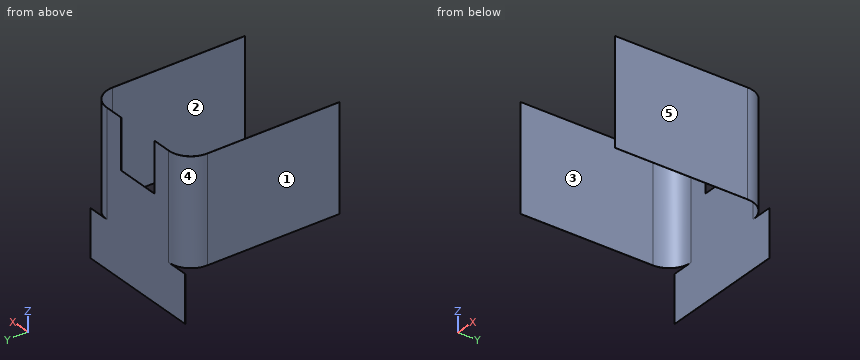
```python
from build123d import *

# Parameters (mm, degrees)
F1_DEPTH = 380
F2_W     = 80
F2_H     = 180
F2_H_2   = 115.651754
F3_DEPTH = 25.4
F4_W     = 230
F4_H     = 170
F5_DEPTH = 0.6


with BuildPart() as f1:
    # F0 (on Top) → F1 (new body)
    with BuildSketch(Plane.XY):
        with BuildLine():
            Line((150, 0), (0, 0))
            Line((0, 0), (-150, 0))
            ThreePointArc((-150, 0), (-206.568542, -23.431458), (-230, -80))
            Line((-230, -80), (-230, -560))
            Line((-230, -560), (-229.4, -560))
            Line((-229.4, -560), (-229.4, -80))
            ThreePointArc((-229.4, -80), (-206.144278, -23.855722), (-150, -0.6))
            Line((-150, -0.6), (0, -0.6))
            Line((0, -0.6), (150, -0.6))
            ThreePointArc((150, -0.6), (206.144278, -23.855722), (229.4, -80))
            Line((229.4, -80), (229.4, -560))
            Line((229.4, -560), (230, -560))
            Line((230, -560), (230, -80))
            ThreePointArc((230, -80), (206.568542, -23.431458), (150, 0))
        make_face()
    extrude(amount=F1_DEPTH)

    # F2 (on face) → F3 (cut)
    with BuildSketch(Plane.XZ.offset(0.6)):
        with Locations((-40, 290)):
            Rectangle(F2_W, F2_H)
        with Locations((40, 290)):
            Rectangle(F2_W, F2_H)
        with Locations((40, 437.825877)):
            Rectangle(F2_W, F2_H_2)
        with Locations((-40, 437.825877)):
            Rectangle(F2_W, F2_H_2)
    extrude(amount=-F3_DEPTH, mode=Mode.SUBTRACT)

    # F4 (on Front) → F5 (join)
    with BuildSketch(Plane.XZ):
        with Locations((115, -85)):
            Rectangle(F4_W, F4_H)
        with Locations((-115, -85)):
            Rectangle(F4_W, F4_H)
    extrude(amount=F5_DEPTH)


solid = f1.part
```
Work out the finished part from the listing and answer in its coordinate system (mm). Face numbers are marked on the shaded views. A direction names the side the tool comes from. Coordinates: 2 decimals unless noted, no trailing zeros. Write each loop counter-clockwise with the first axis right and the second up, starting at its lowest first coordinate (ties: lowest second). Pieces come first, ordered by that corner, then holes.
Q1. Determine the mould class of the marked faces 3, 4 and 5 for opening direction X: released by +X, released by -X, zero draft, split by the parting line, or undercut.
Q2. A cutting plane is placed at D-D, the plane x = -137.5. Give the vertices of the cut face in (y, z), then the cut area to 3 significant figures.
Q3. Which of the six approach directions +Z, -Z, +X, -X, +Y, -Y give full straight-line access (tool end or side, diameter ignored) to the marked faces 1 and 2?
Q4. A cutting plane is placed at C-C, the plane z = 149. Give the vertices of the cut face in (x, y), then the cut area to 3 significant figures.
Q5. Find the intervals of material crossed by line 1 (X direction, y = -85, z = 202); line 2 (Y direction, x = -71.5, z = 35); line 3 (Y direction, x = 182, z = 33.5), in increasing order.
Q6. A cutting plane is placed at A-A, the plane z = 342. Give the vertices of the cut face in (x, y), then the cut area to 3 significant figures.
Q7. Each of these flat-tipped pins is pushed along its axis until it touches: pin 1 Ø0.5 at (x, y) = (-187, -0.5) entering from +Z; pin 2 Ø0.7 at (x, y) = (21, -0.5) entering from +Z. Where does it stop, or does it pass through?
Q8. A cutting plane is placed at B-B, the plane y = -190. Give the vertices of the cut face in (x, z), then the cut area to 3 significant figures.
Findings below:
1. face 3: undercut
1. face 4: released by -X
1. face 5: released by +X
2. outline: (-0.6, -170) - (0, -170) - (0, 380) - (-0.6, 380) - close
2. area: 330 mm2
3. face 1: +Z, -Z, -X, +Y, -Y
3. face 2: +Z, -Z, -Y
4. outline: (-230, -560) - (-229.4, -560) - (-229.4, -80) arc R79.4 cw to (-150, -0.6) - (150, -0.6) arc R79.4 cw to (229.4, -80) - (229.4, -560) - (230, -560) - (230, -80) arc R80 ccw to (150, 0) - (-150, 0) arc R80 ccw to (-230, -80) - close
4. area: 906 mm2
5. line 1: x = -230 to -229.4, 229.4 to 230
5. line 2: y = -0.6 to 0
5. line 3: y = -7.33 to -6.68
6. outline: (-230, -560) - (-229.4, -560) - (-229.4, -80) arc R79.4 cw to (-150, -0.6) - (-80, -0.6) - (-80, 0) - (-150, 0) arc R80 ccw to (-230, -80) - close; (80, -0.6) - (150, -0.6) arc R79.4 cw to (229.4, -80) - (229.4, -560) - (230, -560) - (230, -80) arc R80 ccw to (150, 0) - (80, 0) - close
6. area: 810 mm2
7. pin 1: stops at z = 0
7. pin 2: stops at z = 200
8. outline: (-230, 0) - (-229.4, 0) - (-229.4, 380) - (-230, 380) - close; (229.4, 0) - (230, 0) - (230, 380) - (229.4, 380) - close
8. area: 456 mm2
